from build123d import *

# Parameters (mm, degrees)
PAD_DEPTH = 5


with BuildPart() as part:
    # Sketch → Pad (new body)
    with BuildSketch(Plane.XZ):
        Polygon((16.809578, 52.051549), (59.849419, 52.051549), (52.451943, 8.978119), (76.707435, 8.978119), (56.599094, -29.48042), (72.248703, -29.48042), (34.023357, -73.176758), (36.926517, -28.123772), (17.951936, -28.123772), (36.134954, 6.652457), (9.012691, 6.652457), align=None)
    extrude(amount=PAD_DEPTH)


solid = part.part
Verification items for the finished model (mm, model axes). A direction names the side the tool comes from. Give positions to 0.01 mm unless a question says otherwise; leave off trailing zeros. Loops run counter-clockwise (first coordinate to the right, second up) from the corner with the lowest first, then second, coordinate; pieces in that order, holes last.
1) Sectioned sample at D-D, the plane x = 66. Enter the section's corners in (y, z), then the cut area to 3 significant figures.
2) Sectioned sample at C-C, the plane z = -47. Enter the section's corners in (x, y).
3) Set-up check for faces 1 (the flat face through (12.857, -2.465, 29.034)), 2 (the flat face through (35.455, -2.465, -50.966)), 3 (the flat face through (56.2, -2.5, 30.8)): record each of +Z, -Z, +X, -X, +Y, -Y from which the full face is reachable in a straight line by a thin tool's end or side.
4) Sectioned sample at A-A, the plane y = -1.05. Enter the section's corners in (x, z), then the cut area to 3 significant figures.
5) Thickness scan on line 1 along Z through (x, y) = (65, -3.05); line 2 along Z through (x, y) = (20, -3.05); line 3 along X through (y, z) = (-4.55, 32). Record the ranges inside material, lowest first.
6) Draft check along Z on faces 4 (the flat face through (38, -2, 52.052)), 5 (the flat face through (26.916, -2.465, -10.979)), 6 (the flat face through (23, -2, 6.652)), 7 (the flat face through (43, 0, 4)). Enter one of: pulls with the +Z half, pulls with the -Z half, needs draft (parallel to the pull), parting line crosses it, or undercut.
7) Sectioned sample at B-B, the plane x = 21. Enter the section's corners in (y, z), then the cut area to 3 significant figures.
8) Depth check by flat-ended pin: pin 1 Ø2.5 at (x, y) = (21, -2.5) entering from -Z; pin 2 Ø6 at (x, z) = (59, 19.5) entering from -Y. Enter the tip coordinate at first touch or a pass-through.
Answers:
1. outline: (-5, -36.62) - (0, -36.62) - (0, -29.48) - (-5, -29.48) - close; (-5, -11.5) - (0, -11.5) - (0, 8.98) - (-5, 8.98) - close
1. area: 138 mm2
2. outline: (35.71, -5) - (56.92, -5) - (56.92, 0) - (35.71, 0) - close
3. face 1: +Z, -X, +Y, -Y
3. face 2: -X, +Y, -Y
3. face 3: +X, +Y, -Y
4. outline: (9.01, 6.65) - (36.13, 6.65) - (17.95, -28.12) - (36.93, -28.12) - (34.02, -73.18) - (72.25, -29.48) - (56.6, -29.48) - (76.71, 8.98) - (52.45, 8.98) - (59.85, 52.05) - (16.81, 52.05) - close
4. area: 4,180 mm2
5. line 1: z = -37.77 to -29.48, -13.41 to 8.98
5. line 2: z = -28.12 to -24.21, 6.65 to 52.05
5. line 3: x = 13.37 to 56.41
6. face 4: pulls with the +Z half
6. face 5: undercut
6. face 6: undercut
6. face 7: needs draft
7. outline: (-5, -28.12) - (0, -28.12) - (0, -22.29) - (-5, -22.29) - close; (-5, 6.65) - (0, 6.65) - (0, 52.05) - (-5, 52.05) - close
7. area: 256 mm2
8. pin 1: stops at z = -28.12
8. pin 2: passes through
